```python
from build123d import *

# Parameters (mm, degrees)
BOSS_EXTRUDE1_DEPTH = 90
SKETCH2_W           = 7
SKETCH2_H           = 2
BOSS_EXTRUDE2_DEPTH = 5
BOSS_EXTRUDE3_DEPTH = 8
BOSS_EXTRUDE4_DEPTH = 8


with BuildPart() as part:
    # Sketch1 → Boss-Extrude1 (new body)
    with BuildSketch(Plane(origin=(0, 0, 0), x_dir=(1, 0, 0), z_dir=(0, 1, 0))):
        Polygon((-1.154700538, 2), (-2.309401077, 0), (-1.154700538, -2), (1.154700538, -2), (2.309401077, 0), (1.154700538, 2), align=None)
    extrude(amount=BOSS_EXTRUDE1_DEPTH)

    # Sketch2 → Boss-Extrude2 (add)
    with BuildSketch(Plane(origin=(0, 90, 0), x_dir=(1, 0, 0), z_dir=(0, 1, 0))):
        Rectangle(SKETCH2_W, SKETCH2_H)
    extrude(amount=-BOSS_EXTRUDE2_DEPTH)

    # Sketch3 → Boss-Extrude3 (add)
    with BuildSketch(Plane(origin=(0, 0, 0), x_dir=(0, 0, -1), z_dir=(1, 0, 0))):
        Polygon((-1.5, 6), (-0.5, 6), (1.5, 0), (0.5, 0), align=None)
    extrude(amount=BOSS_EXTRUDE3_DEPTH)

    # Sketch4 → Boss-Extrude4 (add)
    with BuildSketch(Plane(origin=(0, 0, 0), x_dir=(0, 0, -1), z_dir=(1, 0, 0))):
        Polygon((1.5, 6), (0.5, 6), (-1.5, 0), (-0.5, 0), align=None)
    extrude(amount=-BOSS_EXTRUDE4_DEPTH)


solid = part.part
```
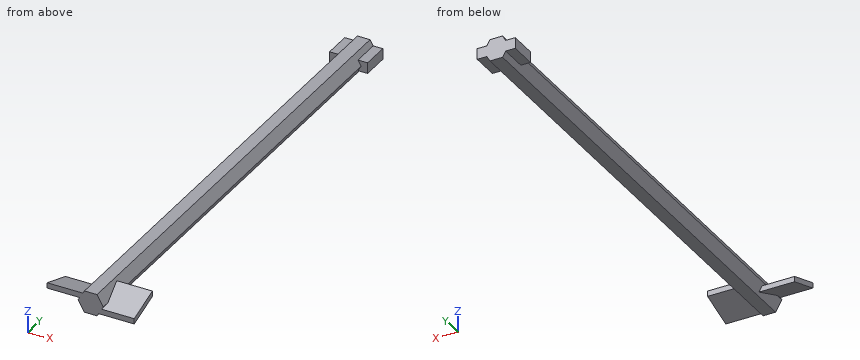
The model under review builds one solid part; all positions refer to its coordinate system, in mm. Coordinates: 2 decimals unless noted, no trailing zeros. Write each loop counter-clockwise with the first axis right and the second up, starting at its lowest first coordinate (ties: lowest second). Pieces come first, ordered by that corner, then holes.
1) To check wall thickness, follow probe 1 along X at (y, z) = (25, 1); probe 2 along X at (y, z) = (52, -0.8); probe 3 along Z at (x, y) = (1.25, 34). State the ranges of each line that lie inside material, in increasing order.
2) We need section B-B on x = 5.25. State the section outline as (y, z) points, then the cut area to 3 significant figures.
3) Clearance check with flat-ended pins moving along their axes: pin 1 Ø1.4 at (x, y) = (2.5, 86.5) entering from -Z; pin 2 Ø2 at (x, y) = (5, 17.5) entering from +Z; pin 3 Ø1.6 at (y, z) = (88, 0) entering from +X; pin 4 Ø8 at (x, y) = (3.5, 60) entering from -Z. State where each tip first meets the part, or that it passes through.
4) We need section A-A on y = 76. State the section outline as (x, z) points.
Answer list:
1. probe 1: x = -1.73 to 1.73
1. probe 2: x = -1.85 to 1.85
1. probe 3: z = -1.83 to 1.83
2. outline: (0, -1.5) - (6, 0.5) - (6, 1.5) - (0, -0.5) - close
2. area: 6.00 mm2
3. pin 1: stops at z = -1
3. pin 2: passes through
3. pin 3: stops at x = 3.5
3. pin 4: stops at z = -2
4. outline: (-2.31, 0) - (-1.15, -2) - (1.15, -2) - (2.31, 0) - (1.15, 2) - (-1.15, 2) - close
